from build123d import *

# Parameters (mm, degrees)
SKETCH1_W           = 20
SKETCH1_H           = 16
SKETCH1_W_2         = 3
SKETCH1_H_2         = 13
BOSS_EXTRUDE1_DEPTH = 4.5
SKETCH2_W           = 9.5
SKETCH2_H           = 16
SKETCH2_W_2         = 3
SKETCH2_H_2         = 13
BOSS_EXTRUDE2_DEPTH = 5.5
FILLET1_R           = 2
FILLET2_R           = 0.5
FILLET3_R           = 0.25


with BuildPart() as part:
    # Sketch1 → Boss-Extrude1 (new body)
    with BuildSketch(Plane(origin=(0, 0, 0), x_dir=(1, 0, 0), z_dir=(0, 1, 0))):
        with Locations((10, -8)):
            Rectangle(SKETCH1_W, SKETCH1_H)
        with Locations((10, -8)):
            Rectangle(SKETCH1_W_2, SKETCH1_H_2, mode=Mode.SUBTRACT)
    extrude(amount=BOSS_EXTRUDE1_DEPTH)

    # Sketch2 → Boss-Extrude2 (add)
    with BuildSketch(Plane(origin=(0, 4.5, 0), x_dir=(1, 0, 0), z_dir=(0, 1, 0))):
        with Locations((10, -8)):
            Rectangle(SKETCH2_W, SKETCH2_H)
        with Locations((10, -8)):
            Rectangle(SKETCH2_W_2, SKETCH2_H_2, mode=Mode.SUBTRACT)
    extrude(amount=BOSS_EXTRUDE2_DEPTH)

    # Fillet1
    fillet1_edges = [part.edges().sort_by_distance(p)[0] for p in [
        (5.25, 4.5, 8),
        (14.75, 4.5, 8),
    ]]
    fillet(fillet1_edges, radius=FILLET1_R)

    # Fillet2
    fillet2_edges = [part.edges().sort_by_distance(p)[0] for p in [
        (20, 4.5, 8),
        (18.375, 4.5, 0),
        (10, 10, 16),
        (10, 10, 0),
        (5.25, 8.25, 0),
        (5.25, 8.25, 16),
        (14.75, 8.25, 16),
        (14.75, 8.25, 0),
        (0, 4.5, 8),
        (1.625, 4.5, 0),
        (18.375, 4.5, 16),
        (4.664213562, 5.085786438, 16),
        (4.664213562, 5.085786438, 0),
        (15.335786438, 5.085786438, 0),
        (15.335786438, 5.085786438, 16),
        (1.625, 4.5, 16),
    ]]
    fillet(fillet2_edges, radius=FILLET2_R)

    # Fillet3
    fillet3_edges = [part.edges().sort_by_distance(p)[0] for p in [
        (8.5, 5, 1.5),
        (8.5, 5, 14.5),
        (11.5, 5, 14.5),
        (11.5, 5, 1.5),
    ]]
    fillet(fillet3_edges, radius=FILLET3_R)


solid = part.part
The listing builds one solid part. Answer for the finished solid, in the listing's coordinates (mm). A direction names the side the tool comes from. Give positions to 0.01 mm unless a question says otherwise; leave off trailing zeros. Order: outer loops, then holes, each group sorted by start corner. A loop starts at its lowest first (then second) coordinate and runs counter-clockwise, first axis right, second up. Notation, with made-up numbers: (-37.5, 88.25) - (5.5, 88.25) arc R13 cw to (5.5, 95.25) - close; hole circle Ø2 at (28.25, 83.5). An arc over 180 degrees is marked (long way). Answer as CSV lines item,"result".
Q1. A cutting plane is placed at A-A, the plane y = 2.25. Determine the outline of the cut face in (x, z), and give its area (3 significant figures).
Answer key:
outline,"(0, 0) - (20, 0) - (20, 16) - (0, 16) - close; hole (8.5, 1.75) arc R0.25 ccw to (8.75, 1.5) - (11.25, 1.5) arc R0.25 ccw to (11.5, 1.75) - (11.5, 14.25) arc R0.25 ccw to (11.25, 14.5) - (8.75, 14.5) arc R0.25 ccw to (8.5, 14.25) - close"
area,"281 mm^2"
Q2. Each of these flat-tipped pins is pushed along its axis until it touches: pin 1 Ø0.8 at (x, z) = (1.5, 5) entering from +Y; pin 2 Ø4 at (x, y) = (5.5, 3) entering from -Z; pin 3 Ø3 at (y, z) = (8.5, 7) entering from +X; pin 4 Ø1.8 at (y, z) = (9, 11) entering from -X. Where does it stop, or does it pass through?
Answer key:
pin 1,"stops at y = 4.5"
pin 2,"stops at z = 0"
pin 3,"stops at x = 14.75"
pin 4,"stops at x = 5.25"
Q3. Which of the six approach directions +Z, -Z, +X, -X, +Y, -Y give full straight-line access (tool end or side, diameter ignored) to faces 4 (the face through (14.75, 8, 8)), 5 (the face through (2, 4.5, 8)), 6 (the face through (10, 5, 1.5))?
Answer key:
face 4,"+Z, -Z, +X, +Y"
face 5,"+Z, -Z, -X, +Y"
face 6,"+Y, -Y"
Q4. Determine the mould class of faces 1 (the face through (10, 4, 0)), 2 (the face through (4.68, 5.1, 7.9)), 3 (the face through (8.5, 5, 8)) for opening direction Z: pulls with the +Z half, pulls with the -Z half, needs draft (parallel to the pull), parting line crosses it, or undercut.
Answer key:
face 1,"pulls with the -Z half"
face 2,"needs draft"
face 3,"undercut"
Q5. A cutting plane is placed at D-D, the plane z = 1.25. Determine the outline of the cut face in (x, y), and give its area (3 significant figures).
Answer key:
outline,"(0, 0) - (20, 0) - (20, 4) arc R0.5 ccw to (19.5, 4.5) - (16.75, 4.5) arc R2 cw to (14.75, 6.5) - (14.75, 10) - (5.25, 10) - (5.25, 6.5) arc R2 cw to (3.25, 4.5) - (0.5, 4.5) arc R0.5 ccw to (0, 4) - close"
area,"144 mm^2"
Q6. A cutting plane is placed at C-C, the plane x = 11. Determine the outline of the cut face in (y, z), and give its area (3 significant figures).
Answer key:
outline,"(0, 0) - (9.5, 0) arc R0.5 ccw to (10, 0.5) - (10, 1.5) - (0, 1.5) - close; (0, 14.5) - (10, 14.5) - (10, 15.5) arc R0.5 ccw to (9.5, 16) - (0, 16) - close"
area,"29.9 mm^2"
Q7. A cutting plane is placed at B-B, the plane z = 5.5. Determine the outline of the cut face in (x, y), and give its area (3 significant figures).
Answer key:
outline,"(0, 0) - (8.5, 0) - (8.5, 10) - (5.25, 10) - (5.25, 6.5) arc R2 cw to (3.25, 4.5) - (0.5, 4.5) arc R0.5 ccw to (0, 4) - close; (11.5, 0) - (20, 0) - (20, 4) arc R0.5 ccw to (19.5, 4.5) - (16.75, 4.5) arc R2 cw to (14.75, 6.5) - (14.75, 10) - (11.5, 10) - close"
area,"114 mm^2"
Q8. Straight lines are drawn through the part: L1, parallel to X at y = 1, z = 13.25; L2, parallel to Z at x = 9, y = 9; L3, parallel to X at y = 8.75, z = 11.75. For each, find the intervals that lie inside material, in ascending order.
Answer key:
L1,"x = 0 to 8.5, 11.5 to 20"
L2,"z = 0 to 1.5, 14.5 to 16"
L3,"x = 5.25 to 8.5, 11.5 to 14.75"
